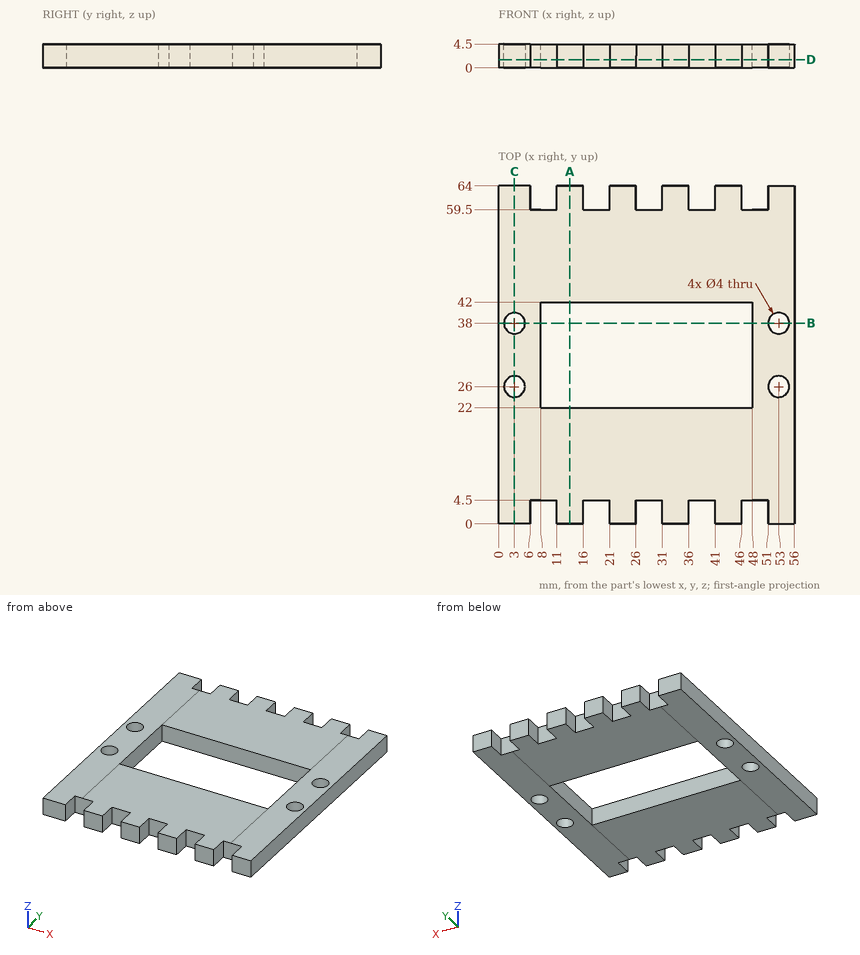
The drawing under review shows one solid part. Ordinate dimensions are in mm from its lowest x, y, z. Give positions to 0.01 mm unless a question says otherwise; leave off trailing zeros. Write each loop counter-clockwise with the first axis right and the second up, starting at its lowest first coordinate (ties: lowest second). Pieces come first, ordered by that corner, then holes. Notation, with made-up numbers: (28.5, -8.75) - (82.5, -8.75) arc R17 ccw to (82.5, 14.25) - close; hole circle Ø5 at (-4.5, 76). An arc over 180 degrees is marked (long way). Answer in a Markdown table with one row per item. Add a question column.
1. Insertion check: P1, Ø2.5, axis at x = 48.5, z = 3, coming from the +Y side. The pin has a flat end and moves straight along its axis. Give the tip position at first contact, or say it passes through.
2. We need section B-B on y = 38. Write out the cut boundary in (x, z), then the cut area to 3 significant figures.
3. We need section A-A on x = 13.5. Write out the cut boundary in (y, z), then the cut area to 3 significant figures.
4. We need section D-D on z = 1.55. State how many separate pieces and enclosed holes the cut face has, then the cut area to 3 significant figures.
5. Wall thickness on line 1 along Y through (x, z) = (53, 3.5); line 2 along X through (y, z) = (4, 0.25); line 3 along X through (y, z) = (39, 3.3): over which ranges is each line inside the solid? List them lowest first. Write a range as [from, to].
6. We need section C-C on x = 3. Write out the cut boundary in (y, z), then the cut area to 3 significant figures.
Ans:
| question | item | result |
|---|---|---|
| 1 | P1 | stops at y = 59.5 |
| 2 | outline | (0, 0) - (1, 0) - (1, 4.5) - (0, 4.5) - close; (5, 0) - (8, 0) - (8, 4.5) - (5, 4.5) - close; (48, 0) - (51, 0) - (51, 4.5) - (48, 4.5) - close; (55, 0) - (56, 0) - (56, 4.5) - (55, 4.5) - close |
| 2 | area | 36.0 mm^2 |
| 3 | outline | (0, 0) - (22, 0) - (22, 4.5) - (0, 4.5) - close; (42, 0) - (64, 0) - (64, 4.5) - (42, 4.5) - close |
| 3 | area | 198 mm^2 |
| 4 | separate pieces | 1 |
| 4 | enclosed holes | 5 |
| 4 | area | 2,510 mm^2 |
| 5 | line 1 | y = [0, 24], [28, 36], [40, 64] |
| 5 | line 2 | x = [0, 6], [11, 16], [21, 26], [31, 36], [41, 46], [51, 56] |
| 5 | line 3 | x = [0, 1.27], [4.73, 8], [48, 51.27], [54.73, 56] |
| 6 | outline | (0, 0) - (24, 0) - (24, 4.5) - (0, 4.5) - close; (28, 0) - (36, 0) - (36, 4.5) - (28, 4.5) - close; (40, 0) - (64, 0) - (64, 4.5) - (40, 4.5) - close |
| 6 | area | 252 mm^2 |
